Drawing for the job (mm, zero at the part's lowest x, y, z). Give positions to 0.01 mm unless a question says otherwise; leave off trailing zeros. Loops run counter-clockwise (first coordinate to the right, second up) from the corner with the lowest first, then second, coordinate; pieces in that order, holes last. Notation, with made-up numbers: (-8, 38) -> (13, 38) arc R10 ccw to (13, 44) -> close; hole circle Ø9 at (72.5, 26.5). An arc over 180 degrees is marked (long way). Write item = value, one per line.
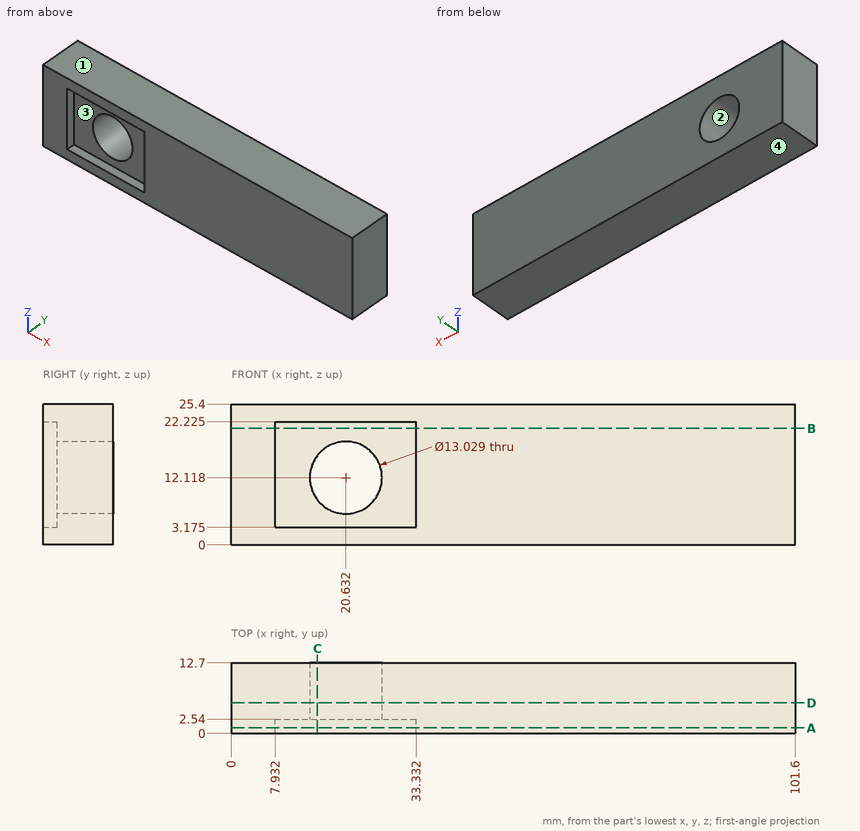
1) Pull direction Z, two halves, no side cores. Call the marked faces 1, 2, 3 and 4: pulls with the +Z half, pulls with the -Z half, needs draft (parallel to the pull), parting line crosses it, or undercut.
Resolved:
face_1 = pulls with the +Z half
face_2 = undercut
face_3 = undercut
face_4 = pulls with the -Z half
2) Slice it at A-A, the plane y = 1. List the corners of the cut face in (x, z) (3 decimals), and give its area (3 significant figures).
Resolved:
outline = (0, 0) -> (101.6, 0) -> (101.6, 25.4) -> (0, 25.4) -> close; hole (7.932, 3.175) -> (33.332, 3.175) -> (33.332, 22.225) -> (7.932, 22.225) -> close
area = 2,100 mm²
3) Slice it at C-C, the plane x = 15.5. List the corners of the cut face in (y, z) (1 decimal).
Resolved:
outline = (0, 0) -> (12.7, 0) -> (12.7, 8.1) -> (2.5, 8.1) -> (2.5, 3.2) -> (0, 3.2) -> close; (0, 22.2) -> (2.5, 22.2) -> (2.5, 16.1) -> (12.7, 16.1) -> (12.7, 25.4) -> (0, 25.4) -> close
4) Slice it at D-D, the plane y = 5.5. List the corners of the cut face in (x, z).
Resolved:
outline = (0, 0) -> (101.6, 0) -> (101.6, 25.4) -> (0, 25.4) -> close; hole circle Ø13.03 at (20.63, 12.12)
5) Drill centre lines: line 1 along X through (y, z) = (2.25, 5.25); line 2 along Y through (x, z) = (27, 15); line 3 along X through (y, z) = (11, 18). Where is each one in solid material? Low to high. Write a range as [from, to].
Resolved:
line_1 = [0, 7.93], [33.33, 101.6]
line_2 = [2.54, 12.7]
line_3 = [0, 17.83], [23.43, 101.6]
6) Slice it at B-B, the plane z = 21. List the corners of the cut face in (x, y).
Resolved:
outline = (0, 0) -> (7.93, 0) -> (7.93, 2.54) -> (33.33, 2.54) -> (33.33, 0) -> (101.6, 0) -> (101.6, 12.7) -> (0, 12.7) -> close
